Could you check a few things on this model? Use its own coordinates, in mm. A direction names the side the tool comes from. Round coordinates to 2 decimals unless told otherwise and drop trailing zeros. Loops run counter-clockwise (first coordinate to the right, second up) from the corner with the lowest first, then second, coordinate; pieces in that order, holes last. Notation, with made-up numbers: (10, 69) - (19, 69) arc R23 cw to (19, 83) - close; hole circle Ø7 at (-37.5, -28.75). An arc over 180 degrees is marked (long way). Put each result on its own line as item: value. Start each with the question number.
from build123d import *

# Parameters (mm, degrees)
EXTRUDE_1_DEPTH               = 80
CUT_EXTRUDE_1_DEPTH           = 74
HOLE_WIZARD_2_05_2_05_1_D     = 2.05
HOLE_WIZARD_2_05_2_05_1_DEPTH = 6
HOLE_WIZARD_1_6_1_6_1_D       = 1.6
HOLE_WIZARD_1_6_1_6_1_DEPTH   = 5.2
HOLE_WIZARD_1_6_1_6_1_TIP     = 0.480688495
HOLE_WIZARD_M2_1_D            = 2.4
HOLE_WIZARD_M2_1_DEPTH        = 6
HOLE_WIZARD_M2_1_CBORE_D      = 4.5
HOLE_WIZARD_M2_1_CBORE_DEPTH  = 2
HOLE_WIZARD_1_D               = 5
HOLE_WIZARD_1_DEPTH           = 80
HOLE_WIZARD_1_CBORE_D         = 11
HOLE_WIZARD_1_CBORE_DEPTH     = 2.2
FILLET_1_R                    = 20
FILLET_2_R                    = 26


with BuildPart() as part:
    # 스케치1 → 보스-돌출1 (new body)
    with BuildSketch(Plane.XZ):
        with BuildLine():
            Line((-25, -31.224989992), (-25, -50))
            Line((-25, -50), (25, -50))
            Line((25, -50), (25, -31.224989992))
            ThreePointArc((25, -31.224989992), (0, 40), (-25, -31.224989992))
        make_face()
    extrude(amount=-EXTRUDE_1_DEPTH)

    # 스케치2 → 컷-돌출1 (cut)
    with BuildSketch(Plane(origin=(0, 80, 0), x_dir=(-1, 0, 0), z_dir=(0, 1, 0))):
        with BuildLine():
            Line((-19, -44), (19, -44))
            Line((19, -44), (19, -28.19574436))
            ThreePointArc((19, -28.19574436), (0, 34), (-19, -28.19574436))
            Line((-19, -28.19574436), (-19, -44))
        make_face()
    extrude(amount=-CUT_EXTRUDE_1_DEPTH, mode=Mode.SUBTRACT)

    # Ø2.05 (2.05) 지름 구멍1
    with Locations(Plane(origin=(0, 0, -50), x_dir=(-1, 0, 0), z_dir=(0, 0, -1))):
        with Locations((-14.666776399, 50), (-14.666776399, 30), (14.666776399, 50), (14.666776399, 30)):
            Hole(HOLE_WIZARD_2_05_2_05_1_D / 2, depth=HOLE_WIZARD_2_05_2_05_1_DEPTH)

    # Ø1.6 (1.6) 지름 구멍1
    with Locations(Plane(origin=(0, 80, 0), x_dir=(1, 0, 0), z_dir=(0, 1, 0))):
        with Locations((0, 47), (-37, 0), (37, 0), (0, -37)):
            Hole(HOLE_WIZARD_1_6_1_6_1_D / 2, depth=HOLE_WIZARD_1_6_1_6_1_DEPTH)
            with Locations((0, 0, -(HOLE_WIZARD_1_6_1_6_1_DEPTH + HOLE_WIZARD_1_6_1_6_1_TIP / 2))):  # 118° drill point
                Cone(0, HOLE_WIZARD_1_6_1_6_1_D / 2, HOLE_WIZARD_1_6_1_6_1_TIP, mode=Mode.SUBTRACT)

    # M2 육각 머리 작은 나사용 카운터보어1
    with Locations(Plane(origin=(0, 6, 0), x_dir=(1, 0, 0), z_dir=(0, 1, 0))):
        with Locations((0, 8), (5.656854249, 5.656854249), (8, 0), (5.656854249, -5.656854249), (0, -8), (-5.656854249, -5.656854249), (-8, 0), (-5.656854249, 5.656854249)):
            CounterBoreHole(HOLE_WIZARD_M2_1_D / 2, HOLE_WIZARD_M2_1_CBORE_D / 2, HOLE_WIZARD_M2_1_CBORE_DEPTH, depth=HOLE_WIZARD_M2_1_DEPTH)

    # 구멍1
    with Locations(Plane(origin=(0, 0, 0), x_dir=(-1, 0, 0), z_dir=(0, -1, 0))):
        with Locations((0, 0)):
            CounterBoreHole(HOLE_WIZARD_1_D / 2, HOLE_WIZARD_1_CBORE_D / 2, HOLE_WIZARD_1_CBORE_DEPTH, depth=HOLE_WIZARD_1_DEPTH)

    # 필렛1
    fillet_1_edges = [part.edges().sort_by_distance(p)[0] for p in [
        (25, 40, -31.224989992),
        (-25, 40, -31.224989992),
    ]]
    fillet(fillet_1_edges, radius=FILLET_1_R)

    # 필렛2
    fillet_2_edges = [part.edges().sort_by_distance(p)[0] for p in [
        (19, 43, -28.19574436),
        (-19, 43, -28.19574436),
    ]]
    fillet(fillet_2_edges, radius=FILLET_2_R)


solid = part.part
Item 1: Thinking about a two-plate mould opening in X: for faces 1 (the face through (6.856, 1.972, 5.604)), 2 (the face through (19, 44, -42)), 3 (the face through (26.33, 40.56, -32.52)), 4 (the face through (0, 39, -50)), which applies, released by +X, released by -X, zero draft, split by the parting line, or undercut?
Item 2: Suppose I cut it at C-C, the plane x = 22. List the corners of the cut face in (y, z) for me.
Item 3: Will these pins go through, and if not, where does the flat tip stop? P1, Ø2.5, axis at x = 14.67, y = 30, coming from the +Z side; P2, Ø2, axis at x = 4.5, z = 6.5, coming from the +Y side; P3, Ø4, axis at y = 16, z = 11, coming from the -X side.
Item 4: On a 3-axis mill with a long thin cutter (end or side, diameter ignored), from which of +Z, -Z, +X, -X, +Y, -Y can I reach the whole of each face in a straight line? I mean faces 5 (the face through (8, 0, -4)), 6 (the face through (3, 2.2, 0)), 7 (the face through (7, 4, -5)). Say none if no direction works.
Item 5: Suppose I cut it at B-B, the plane z = 23. List the corners of the cut face in (x, y) for me.
Item 6: I need wall thicknesses on line 1 (Z direction, x = 0, y = 78.5); line 2 (Z direction, x = 0, y = 5); line 3 (X direction, y = 60, z = -39). Which ranges of each line are inside material? Lowest first, please. Write a range as from..to.
Item 7: Suppose I cut it at A-A, the plane y = 68. List the corners of the cut face in (x, z) for me.
Numbers:
1. face 1: undercut
1. face 2: undercut
1. face 3: released by +X
1. face 4: zero draft
2. outline: (0, -50) - (80, -50) - (80, -27.56) - (6, -27.56) - (6, 25.92) - (80, 25.92) - (80, 33.41) - (0, 33.41) - close
3. P1: z = 37.68
3. P2: y = 6
3. P3: x = -38.97
4. face 5: +Z, -Z, +X, -X, -Y
4. face 6: -Y
4. face 7: +Y
5. outline: (-32.73, 0) - (32.73, 0) - (32.73, 80) - (25.04, 80) - (25.04, 6) - (-25.04, 6) - (-25.04, 80) - (-32.73, 80) - close
6. line 1: -50..-47.8, -46.2..-44, 34..36.2, 37.8..40
6. line 2: -50..-10.25, -5.75..-2.5, 2.5..5.75, 10.25..40
6. line 3: -25.01..-19.01, 19.01..25.01
7. outline: (-30, -26.46) arc R20 cw to (-25, -39.69) - (-25, -50) - (25, -50) - (25, -39.69) arc R20 cw to (30, -26.46) arc R40 ccw (long way) to start; hole (-25.5, -22.49) arc R26 cw to (-19, -39.69) - (-19, -44) - (19, -44) - (19, -39.69) arc R26 cw to (25.5, -22.49) arc R34 ccw (long way) to start
